Could you check a few things on this model? Use its own coordinates, in mm. A direction names the side the tool comes from. Give positions to 0.01 mm unless a question says otherwise; leave off trailing zeros. Loops run counter-clockwise (first coordinate to the right, second up) from the corner with the lowest first, then second, coordinate; pieces in that order, holes last. Notation, with made-up numbers: (43, -2) -> (64, -2) arc R15 ccw to (64, 10) -> close; hole circle Ø1 at (40, 19). An arc over 180 degrees is marked (long way). Write item = value, one per line. Start each with the question number.
1) I want a section at C-C (z = 5). List the corners of the cut face in (x, y) for me, and give its area (3 significant figures).
2) I want a section at B-B (x = 19). List the corners of the cut face in (y, z) for me, and give its area (3 significant figures).
3) If we mould it in two halves opening along X, with no side actions, what happens to faces 1 (the face through (0.538, 11.816, 4.93)), 2 (the face through (12.372, 20.494, 24.65)), 3 (the face through (-5, 16, 0))? For each: +X half, -X half, draft (parallel to the pull), parting line (faces both ways), or undercut.
4) I want a section at A-A (z = 42). List the corners of the cut face in (x, y) for me, and give its area (3 significant figures).
5) On a 3-axis mill with a long thin cutter (end or side, diameter ignored), from which of +Z, -Z, +X, -X, +Y, -Y can I reach the whole of each face in a straight line? I mean faces 4 (the face through (-11.628, 21.076, 24.65)), 5 (the face through (0, 14, 10)). Say none if no direction works.
6) I need wall thicknesses on probe 1 along Y at (x, z) = (0, 4.5); probe 2 along Z at (x, y) = (-1, 14); probe 3 along Y at (x, z) = (-1, 27.5). Which ranges of each line are inside material? Lowest first, please. Write a range as from..to.
7) I want a section at D-D (y = 8.5). List the corners of the cut face in (x, z) for me.
8) I'm going to push flat-ended pins straight in: pin 1 Ø5.5 at (x, y) = (1, 13) entering from -Z; pin 2 Ø2 at (y, z) = (31.5, 36.5) entering from -X; pin 3 Ø5 at (x, z) = (5.5, 7) entering from +Y; pin 4 Ø1 at (x, z) = (8, 43) entering from +Y. Where does each tip first touch, or does it pass through?
from build123d import *

# Parameters (mm, degrees)
SALIENTE_EXTRUIR2_DEPTH = 50
CROQUIS3_R              = 2.482100889
CORTAR_EXTRUIR1_DEPTH   = 10


with BuildPart() as part:
    # Croquis1 → Saliente-Extruir2 (new body)
    with BuildSketch(Plane.XY):
        Polygon((0.204464985, 41.569219382), (-23.795535015, 0), (24.204464985, 0), align=None)
    extrude(amount=SALIENTE_EXTRUIR2_DEPTH)

    # Croquis3 → Cortar-Extruir1 (cut)
    with BuildSketch(Plane(origin=(0, 0, 0), x_dir=(-1, 0, 0), z_dir=(0, 0, -1))):
        with Locations((0, 14.238722588)):
            Circle(CROQUIS3_R)
    extrude(amount=-CORTAR_EXTRUIR1_DEPTH, mode=Mode.SUBTRACT)


solid = part.part
Answer list:
q1.outline = (-23.8, 0) -> (24.2, 0) -> (0.2, 41.57) -> close; hole circle Ø4.96 at (0, 14.24)
q1.area = 978 mm^2
q2.outline = (0, 0) -> (9.01, 0) -> (9.01, 50) -> (0, 50) -> close
q2.area = 451 mm^2
q3.face_1 = undercut
q3.face_2 = +X half
q3.face_3 = draft
q4.outline = (-23.8, 0) -> (24.2, 0) -> (0.2, 41.57) -> close
q4.area = 998 mm^2
q5.face_4 = +Z, -Z, -X, +Y
q5.face_5 = -Z
q6.probe_1 = 0..11.76, 16.72..41.22
q6.probe_2 = 10..50
q6.probe_3 = 0..39.48
q7.outline = (-18.89, 0) -> (19.3, 0) -> (19.3, 50) -> (-18.89, 50) -> close
q8.pin_1 = 0
q8.pin_2 = -6.19
q8.pin_3 = 36.73
q8.pin_4 = 28.93
